```python
from build123d import *

# Parameters (mm, degrees)
BOSS_EXTRUDE1_DEPTH = 3
CUT_EXTRUDE1_DEPTH  = 10
SKETCH3_W           = 65
SKETCH3_H           = 3
CUT_EXTRUDE2_DEPTH  = 10
FILLET1_START       = -1
FILLET1_DEPTH       = 5
SKETCH4_W           = 3
SKETCH4_H           = 10
CUT_EXTRUDE3_DEPTH  = 10
BOSS_EXTRUDE2_DEPTH = 3
FILLET2_R           = 10


with BuildPart() as part:
    # Sketch1 → Boss-Extrude1 (new body)
    with BuildSketch(Plane.XY):
        with BuildLine():
            add(Edge.make_bspline(
                [(-70, -11.5), (-70, 26.5), (-18, 33.5), (-10, 33.5)],
                knots=[0, 0, 0, 0, 1, 1, 1, 1], degree=3))
            Line((-70, -11.5), (-70, -46.5))
            ThreePointArc((-70, -46.5), (-55.355339059, -81.855339059), (-20, -96.5))
            Line((-20, -96.5), (20, -96.5))
            ThreePointArc((20, -96.5), (55.355339059, -81.855339059), (70, -46.5))
            Line((70, -46.5), (70, -11.5))
            add(Edge.make_bspline(
                [(10, 33.5), (18, 33.5), (70, 26.5), (70, -11.5)],
                knots=[0, 0, 0, 0, 1, 1, 1, 1], degree=3))
            Line((10, 33.5), (-10, 33.5))
        make_face()
    extrude(amount=BOSS_EXTRUDE1_DEPTH)

    # Sketch2 → Cut-Extrude1 (cut)
    with BuildSketch(Plane.XY.offset(3)):
        with BuildLine():
            Line((-22.5, -40), (22.5, -40))
            ThreePointArc((22.5, -40), (29.571067812, -37.071067812), (32.5, -30))
            Line((32.5, -30), (32.5, 5))
            ThreePointArc((32.5, 5), (29.571067812, 12.071067812), (22.5, 15))
            Line((22.5, 15), (-22.5, 15))
            ThreePointArc((-22.5, 15), (-29.571067812, 12.071067812), (-32.5, 5))
            Line((-32.5, 5), (-32.5, -30))
            ThreePointArc((-32.5, -30), (-29.571067812, -37.071067812), (-22.5, -40))
        make_face()
    extrude(amount=-CUT_EXTRUDE1_DEPTH, mode=Mode.SUBTRACT)

    # Sketch3 → Cut-Extrude2 (cut)
    with BuildSketch(Plane.XY.offset(3)):
        with Locations((0, -41.5)):
            Rectangle(SKETCH3_W, SKETCH3_H)
        with BuildLine():
            Line((-26.880912438, -54.126379534), (26.880912438, -54.126379534))
            ThreePointArc((26.880912438, -54.126379534), (42.22301594, -69.468483036), (26.880912438, -84.810586538))
            Line((26.880912438, -84.810586538), (-26.880912438, -84.810586538))
            ThreePointArc((-26.880912438, -84.810586538), (-42.22301594, -69.468483036), (-26.880912438, -54.126379534))
        make_face()
        with BuildLine():
            Line((-39.64451115, -4.103386604), (-39.64451115, -43.425584655))
            ThreePointArc((-39.64451115, -43.425584655), (-50.732081748, -54.513155253), (-61.819652346, -43.425584655))
            Line((-61.819652346, -43.425584655), (-61.819652346, -4.103386604))
            ThreePointArc((-61.819652346, -4.103386604), (-50.732081748, 6.984183994), (-39.64451115, -4.103386604))
        make_face()
        with BuildLine():
            Line((39.64451115, -4.103386604), (39.64451115, -43.425584655))
            ThreePointArc((39.64451115, -43.425584655), (50.732081748, -54.513155253), (61.819652346, -43.425584655))
            Line((61.819652346, -43.425584655), (61.819652346, -4.103386604))
            ThreePointArc((61.819652346, -4.103386604), (50.732081748, 6.984183994), (39.64451115, -4.103386604))
        make_face()
    extrude(amount=-CUT_EXTRUDE2_DEPTH, mode=Mode.SUBTRACT)

    # Fillet1: read off the stored shape, not the designer's step
    # Fillet1 outline → Fillet1 (cut)
    with BuildSketch(Plane.XY.offset(FILLET1_START)):
        with BuildLine():
            ThreePointArc((28.82455532, -40), (27.871092731, -39.301511345), (28.249595746, -38.181818182))
            ThreePointArc((28.249595746, -38.181818182), (25.515113446, -39.534625893), (22.5, -40))
            Line((22.5, -40), (28.82455532, -40))
        make_face()
        with BuildLine():
            ThreePointArc((-28.249595746, -38.181818182), (-27.871092731, -39.301511345), (-28.82455532, -40))
            Line((-28.82455532, -40), (-22.5, -40))
            ThreePointArc((-22.5, -40), (-25.515113446, -39.534625893), (-28.249595746, -38.181818182))
        make_face()
    extrude(amount=FILLET1_DEPTH, mode=Mode.SUBTRACT)

    # Sketch4 → Cut-Extrude3 (cut)
    with BuildSketch(Plane.XY.offset(3)):
        with Locations((0, -48)):
            Rectangle(SKETCH4_W, SKETCH4_H)
    extrude(amount=-CUT_EXTRUDE3_DEPTH, mode=Mode.SUBTRACT)

    # Sketch5 → Boss-Extrude2 (add)
    with BuildSketch(Plane.XY.offset(3)):
        with BuildLine():
            Line((-4, -54.126379534), (4, -54.126379534))
            ThreePointArc((4, -54.126379534), (0, -58.126379534), (-4, -54.126379534))
        make_face()
    extrude(amount=-BOSS_EXTRUDE2_DEPTH)

    # Fillet2
    fillet2_edges = [part.edges().sort_by_distance(p)[0] for p in [
        (4, -54.126379534, 1.5),
        (-4, -54.126379534, 1.5),
    ]]
    fillet(fillet2_edges, radius=FILLET2_R)


solid = part.part
```
Work out the finished part from the listing and answer in its coordinate system (mm). A direction names the side the tool comes from. Coordinates: 2 decimals unless noted, no trailing zeros. Order: outer loops, then holes, each group sorted by start corner. A loop starts at its lowest first (then second) coordinate and runs counter-clockwise, first axis right, second up. Notation, with made-up numbers: (66, 67) - (73, 67) arc R21 ccw to (73, 75) - close; hole circle Ø2 at (78.25, 58.25). An arc over 180 degrees is marked (long way). Answer as a JSON object with one key per item and string values.
1. Consider line 1 (Y direction, x = -7, z = 2.25); line 2 (X direction, y = -23, z = 1.6); line 3 (Y direction, x = 9.5, z = 1.05). Determine where each line is inside the solid, lowest interval first.
Output values:
{"line 1": "y = -96.5 to -84.81, -54.53 to -43, 15 to 33.5", "line 2": "x = -70 to -61.82, -39.64 to -32.5, 32.5 to 39.64, 61.82 to 70", "line 3": "y = -96.5 to -84.81, -54.13 to -43, 15 to 33.5"}
2. Each of these flat-tipped pins is pushed along its axis until it touches: P1, Ø0.9, axis at y = -49, z = 1, coming from the -X side; P2, Ø0.9, axis at x = 10.5, z = 1.5, coming from the +Y side; P3, Ø1.5, axis at y = -51.5, z = 2.5, coming from the +X side; P4, Ø1.5, axis at y = -8, z = 2, coming from the +X side. Where does it stop, or does it pass through?
Output values:
{"P1": "stops at x = -69.96", "P2": "stops at y = 33.5", "P3": "stops at x = 69.82", "P4": "stops at x = 69.91"}
3. Find section A-A on y = -25.5. Determine the outline of the cut face in (x, z).
Output values:
{"outline": "(-70, 0) - (-61.82, 0) - (-61.82, 3) - (-70, 3) - close; (-39.64, 0) - (-32.5, 0) - (-32.5, 3) - (-39.64, 3) - close; (32.5, 0) - (39.64, 0) - (39.64, 3) - (32.5, 3) - close; (61.82, 0) - (70, 0) - (70, 3) - (61.82, 3) - close"}
4. Find section D-D on z = 1.5. Count the separate pieces of the cut face and the enclosed holes in it, plus the area to 3 significant figures.
Output values:
{"separate pieces": "1", "enclosed holes": "4", "area": "7,330 mm²"}
5. Find section B-B on x = 8. Determine the outline of the cut face in (y, z), plus the area to 3 significant figures.
Output values:
{"outline": "(-96.5, 0) - (-84.81, 0) - (-84.81, 3) - (-96.5, 3) - close; (-54.29, 0) - (-43, 0) - (-43, 3) - (-54.29, 3) - close; (15, 0) - (33.5, 0) - (33.5, 3) - (15, 3) - close", "area": "124 mm²"}
6. Find section C-C on y = -78.5. Determine the outline of the cut face in (x, z).
Output values:
{"outline": "(-58.42, 0) - (-39.28, 0) - (-39.28, 3) - (-58.42, 3) - close; (39.28, 0) - (58.42, 0) - (58.42, 3) - (39.28, 3) - close"}
7. A tool of negligible diameter and unlimited length cuts with its end or side. For faces 1 (the face through (31.343, -34.669, 1.521)), 2 (the face through (54.964, -82.242, 1.479)), from which of +Z, -Z, +X, -X, +Y, -Y can it reach the whole face along a straight path? Write none if from no direction.
Output values:
{"face 1": "+Z, -Z", "face 2": "+Z, -Z, +X, -Y"}
